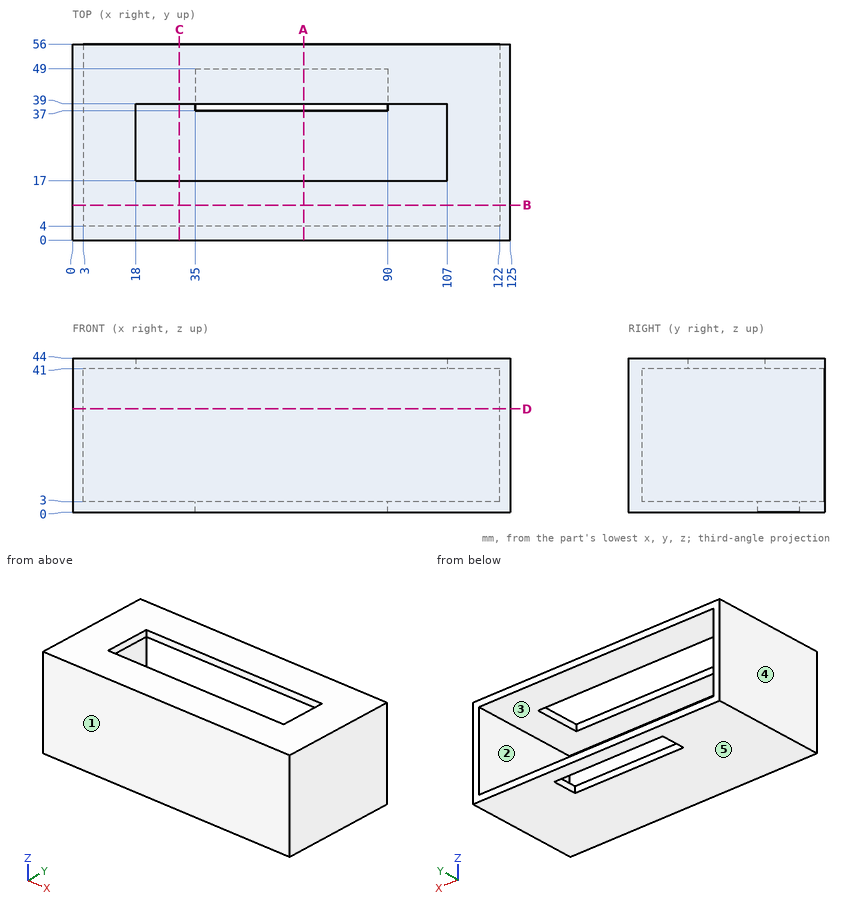
Verification items for this drawing (mm, ordinates from the low corner). A direction names the side the tool comes from. Coordinates: 2 decimals unless noted, no trailing zeros. Loops run counter-clockwise (first coordinate to the right, second up) from the corner with the lowest first, then second, coordinate; pieces in that order, holes last. Notation, with made-up numbers: (-11, -34.5) - (15, -34.5) arc R28 ccw to (15, -9.5) - close; hole circle Ø11 at (34, -24.5). An arc over 180 degrees is marked (long way). Use one line per item in the form item = value. Start each with the question number.
Item 1: Thickness scan on probe 1 along Z at (x, y) = (12.5, 43); probe 2 along X at (y, z) = (27, 36); probe 3 along Z at (x, y) = (49, 46). Record the ranges inside material, lowest first.
Item 2: Tool access check on the marked faces 1 and 2. Record the directions out of +Z, -Z, +X, -X, +Y, -Y that give a thin tool (end or side, any length) a straight path to the whole face; none if there is none.
Item 3: Section check A-A, the plane x = 66. Enter the section's corners in (y, z).
Item 4: Mould release check, pull along Z, two halves, no side actions. Record for the marked faces 3, 4 and 5: +Z half, -Z half, draft (parallel to the pull), parting line (faces both ways), or undercut.
Item 5: Section check D-D, the plane z = 29.5. Enter the section's corners in (x, y).
Item 6: Gauge pin test, flat ends, axial feed: pin 1 (2.5 mm diameter, centred on x = 74.5, z = 1.5, fed in from -Y); pin 2 (12 mm diameter, centred on x = 109, z = 30, fed in from +Y); pin 3 (1 mm diameter, centred on x = 79, y = 19, fed in from +Z). Record the tip position at first contact, or that the pin passes through.
Item 7: Section check B-B, the plane y = 10. Enter the section's corners in (x, z), and give its area (3 significant figures).
Item 8: Section check C-C, the plane x = 30.5. Enter the section's corners in (y, z), and give its area (3 significant figures).
Computed:
q1.probe_1 = 0 to 3, 41 to 44
q1.probe_2 = 0 to 3, 122 to 125
q1.probe_3 = 41 to 44
q2.face_1 = +Z, -Z, +X, -X, -Y
q2.face_2 = +Y
q3.outline = (0, 0) - (37, 0) - (37, 3) - (4, 3) - (4, 41) - (17, 41) - (17, 44) - (0, 44) - close; (39, 41) - (56, 41) - (56, 44) - (39, 44) - close; (49, 0) - (56, 0) - (56, 3) - (49, 3) - close
q4.face_3 = undercut
q4.face_4 = draft
q4.face_5 = -Z half
q5.outline = (0, 0) - (125, 0) - (125, 56) - (122, 56) - (122, 4) - (3, 4) - (3, 56) - (0, 56) - close
q6.pin_1 = 0
q6.pin_2 = 4
q6.pin_3 = 3
q7.outline = (0, 0) - (125, 0) - (125, 44) - (0, 44) - close; hole (3, 3) - (122, 3) - (122, 41) - (3, 41) - close
q7.area = 978 mm2
q8.outline = (0, 0) - (56, 0) - (56, 3) - (4, 3) - (4, 41) - (17, 41) - (17, 44) - (0, 44) - close; (39, 41) - (56, 41) - (56, 44) - (39, 44) - close
q8.area = 422 mm2
